```python
from build123d import *

# Parameters (mm, degrees)
SKETCH1_W           = 20
SKETCH1_H           = 8
BOSS_EXTRUDE1_DEPTH = 30
SKETCH2_W           = 40
SKETCH2_H           = 40
BOSS_EXTRUDE2_DEPTH = 20
FILLET1_R           = 10


with BuildPart() as part:
    # Sketch1 → Boss-Extrude1 (new body)
    with BuildSketch(Plane.XY):
        with Locations((-20, -4)):
            Rectangle(SKETCH1_W, SKETCH1_H)
    extrude(amount=BOSS_EXTRUDE1_DEPTH)

    # Sketch2 → Boss-Extrude2 (add)
    with BuildSketch(Plane.XY):
        with Locations((-10, 12)):
            Rectangle(SKETCH2_W, SKETCH2_H)
    extrude(amount=-BOSS_EXTRUDE2_DEPTH)

    # Fillet1
    # the kernel refuses this fillet: 10 mm, written as the material it adds along each edge
    with BuildSketch(Plane(origin=(-10, 0, 0), x_dir=(0, 1, 0), z_dir=(-1, 0, 0))) as fillet1_piece_1:
        with BuildLine():
            CenterArc((FILLET1_R, -FILLET1_R), FILLET1_R, 90, 90)
            Line((0, -FILLET1_R), (0, 0))
            Line((0, 0), (FILLET1_R, 0))
        make_face()
    extrude(amount=20)
    # the kernel refuses this fillet: 10 mm, written as the material it takes off along each edge
    with BuildSketch(Plane(origin=(10, 32, 25), x_dir=(-1, 0, 0), z_dir=(0, 0, -1))) as fillet1_2_piece_1:
        with BuildLine():
            CenterArc((FILLET1_R, -FILLET1_R), FILLET1_R, 90, 90)
            Line((0, -FILLET1_R), (0, 0))
            Line((0, 0), (FILLET1_R, 0))
        make_face()
    extrude(amount=70, mode=Mode.SUBTRACT)
    with BuildSketch(Plane(origin=(14.494897428, 0, 30), x_dir=(0, 0, -1), z_dir=(-1, 0, 0))) as fillet1_2_piece_2:
        with BuildLine():
            CenterArc((9.797958971, 10), FILLET1_R, 191.536959033, 78.463040967)
            Line((0, 8), (0, 0))
            Line((0, 0), (9.797958971, 0))
        make_face()
    extrude(amount=68.989794856, mode=Mode.SUBTRACT)


solid = part.part
```
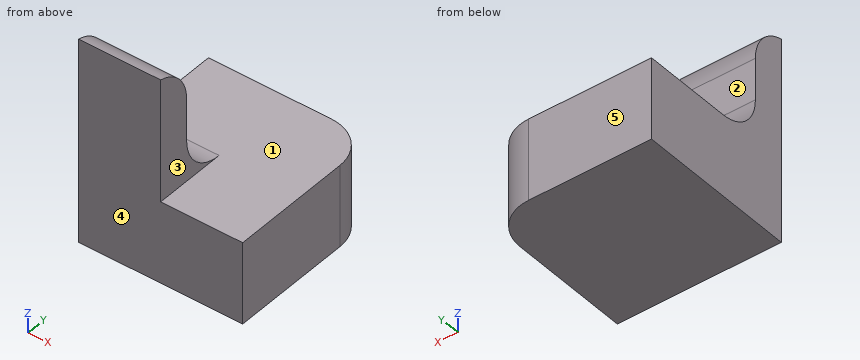
The model under review builds one solid part; all positions refer to its coordinate system, in mm. Face numbers are marked on the shaded views. A direction names the side the tool comes from. Coordinates: 2 decimals unless noted, no trailing zeros. Order: outer loops, then holes, each group sorted by start corner. A loop starts at its lowest first (then second) coordinate and runs counter-clockwise, first axis right, second up. Notation, with made-up numbers: M -28,62.5 L -18,62.5 A20 ccw -18,86.5 Z; hole C 55,31 d9. An arc over 180 degrees is marked long. One line per question, with ' | ' between items.
(1) For probe 1 along Z at (x, y) = (-5.5, 1.5); probe 2 along Y at (x, z) = (-28, 19); probe 3 along Z at (x, y) = (-27.5, -6), list the stretches that pass through material, from the lowest coordinate up. Write a range as from..to.
Geometry results:
probe 1: z = -20..0 | probe 2: y = -8..0 | probe 3: z = -20..29.37
(2) Add section C-C, the plane z = 16. Write out the cut boundary in (x, y).
Geometry results:
outline: M -30,-8 L -10,-8 L -10,0 L -30,0 Z
(3) Add section D-D, the plane y = 11. Write out the cut boundary in (x, z), then the cut area to 3 significant figures.
Geometry results:
outline: M -30,-20 L 10,-20 L 10,0 L -30,0 Z | area: 800 mm²
(4) Add section A-A, the plane x = -27. Write out the cut boundary in (y, z), then the cut area to 3 significant figures.
Geometry results:
outline: M -8,-20 L 32,-20 L 32,0 L 10,0 A10 cw 0,10 L 0,20.2 A10 ccw -8,30 Z | area: 1,040 mm²
(5) Add section B-B, the plane y = 1. Write out the cut boundary in (x, z), then the cut area to 3 significant figures.
Geometry results:
outline: M -30,-20 L 10,-20 L 10,0 L -10,0 L -10,5.64 L -30,5.64 Z | area: 913 mm²
(6) Insertion check: pin 1 (3 mm diameter, centred on x = -1, z = 3, fed in from +Y); pin 2 (12 mm diameter, centred on x = -5, y = 19, fed in from +Z); pin 3 (9 mm diameter, centred on y = 3, z = 21.5, fed in from +X); pin 4 (5 mm diameter, centred on x = -18.5, z = 15.5, fed in from +Y). Each pin has a flat end and moves straight along its axis. Give the tip position at first contact, or say it passes through.
Geometry results:
pin 1: passes through | pin 2: stops at z = 0 | pin 3: stops at x = -10 | pin 4: stops at y = 0
(7) Machinability: for the marked faces 1, 2, 3, 4 and 5, which of the approach directions +Z, -Z, +X, -X, +Y, -Y give a long, thin tool a straight path to every point of the face, cutting with its end or side? Answer none if there is none.
Geometry results:
face 1: +Z, +X, +Y | face 2: +Z, +X, -X, +Y | face 3: +Z, +X, +Y, -Y | face 4: +Z, -Z, +X, -X, -Y | face 5: +Z, -Z, +X, -X, +Y
